CAD build for the part. Positions are in the model's coordinates, mm. A direction names the side the tool comes from. Coordinates: 2 decimals unless noted, no trailing zeros. Loops run counter-clockwise (first coordinate to the right, second up) from the corner with the lowest first, then second, coordinate; pieces in that order, holes last.
1) Saw through at B-B, the plane x = 113.5. Write the cut outline in (y, z), and give its area (3 significant figures).
2) Which spindle directions (+Z, -Z, +X, -X, +Y, -Y) get a long thin tool onto all of the face, cutting with end or side? Do faces 1 (the flat face through (109, 0, -8)), 2 (the flat face through (7, -5.634, -13)), 3 (the flat face through (184.81, 1.84, 1.58)). Say none if no direction does.
3) Saw through at A-A, the plane y = -3.5. Write the cut outline in (x, z), and give its area (3 significant figures).
4) Pin check, flat tips, straight feed: pin 1 Ø0.6 at (x, z) = (161.5, -15) entering from -Y; pin 2 Ø2 at (y, z) = (1, -14.5) entering from +X; pin 3 Ø3.5 at (x, z) = (64.5, -7.5) entering from +Y; pin 4 Ø5 at (x, y) = (129.5, 2.5) entering from +Z. Stop position of each tip, or through.
5) Saw through at C-C, the plane z = -6. Write the cut outline in (x, y).
6) Saw through at D-D, the plane x = 86.5. Write the cut outline in (y, z).
7) Two-plate mould, pull along X, no slides. Class faces 4 (the flat face through (203, -3, -16)), 5 (the flat face through (206, -1, -9)), 6 (the flat face through (15, -2, -10)): +X half, -X half, draft (parallel to the pull), parting line (faces both ways), or undercut.
8) Wall check: line 1 along X through (y, z) = (-1.5, -8.25); line 2 along Z through (x, y) = (152.5, 2.5); line 3 along Y through (x, z) = (93, -15). Give the ranges that are in metal, low to high.
```python
from build123d import *

# Parameters (mm, degrees)
EXTRUDE_PROFILE_DEPTH = 206
SKETCH6_W             = 185
SKETCH6_H             = 5.633658753
AIR_SPACE_DEPTH       = 45
SKETCH7_W             = 12
SKETCH7_H             = 3.530528437
TAB_CUTS_DEPTH        = 8.515248173
SKETCH8_W             = 15.5
SKETCH8_H             = 10
SKETCH8_W_2           = 6.5
CUT_EXTRUDE1_DEPTH    = 2


with BuildPart() as part:
    # Sketch1 → Extrude profile (new body)
    with BuildSketch(Plane(origin=(0, 0, 0), x_dir=(0, 0, -1), z_dir=(1, 0, 0))):
        Polygon((0, 1), (12, 1), (12, 4), (12, 5), (15, 5), (16, 4), (14, 4), (14, 2), (16, 2), (16, -5.633658753), (10.595371114, -5.633658753), (0, 0), (-3.531790371, 1.877886251), (-3.117271585, 2.657482703), align=None)
    extrude(amount=EXTRUDE_PROFILE_DEPTH)

    # Sketch6 → Air space (cut)
    with BuildSketch(Plane(origin=(0, 0, -16), x_dir=(-1, 0, 0), z_dir=(0, 0, -1))):
        with Locations((-107.5, -2.816829377)):
            Rectangle(SKETCH6_W, SKETCH6_H)
    extrude(amount=-AIR_SPACE_DEPTH, mode=Mode.SUBTRACT)

    # Sketch7 → Tab cuts (cut, through all)
    with BuildSketch(Plane(origin=(0, 0.779596452, -0.414518786), x_dir=(1, 0, 0), z_dir=(0, 0.882947593, -0.469471563))):
        with Locations((158.2, -2.234735781)):
            Rectangle(SKETCH7_W, SKETCH7_H)
        with Locations((88.1, -2.234735781)):
            Rectangle(SKETCH7_W, SKETCH7_H)
    extrude(amount=-TAB_CUTS_DEPTH, mode=Mode.SUBTRACT)

    # Sketch8 → Cut-Extrude1 (cut)
    with BuildSketch(Plane(origin=(0, 0, -16), x_dir=(-1, 0, 0), z_dir=(0, 0, -1))):
        with Locations((-198.25, 5)):
            Rectangle(SKETCH8_W, SKETCH8_H)
        with Locations((-70.55, 5)):
            Rectangle(SKETCH8_W_2, SKETCH8_H)
        with Locations((-79.45, 5)):
            Rectangle(SKETCH8_W_2, SKETCH8_H)
    extrude(amount=-CUT_EXTRUDE1_DEPTH, mode=Mode.SUBTRACT)


solid = part.part
```
Data:
1. outline: (0, -16) - (2, -16) - (2, -14) - (4, -14) - (4, -16) - (5, -15) - (5, -12) - (1, -12) - (1, 0) - (2.66, 3.12) - (1.88, 3.53) - (0, 0) - close
1. area: 30.8 mm2
2. face 1: +Z, -Z, -Y
2. face 2: +Z, -Z, +X, -X, -Y
2. face 3: +X, -X, +Y
3. outline: (0, -16) - (15, -16) - (15, -6.58) - (0, -6.58) - close; (200, -16) - (206, -16) - (206, -6.58) - (200, -6.58) - close
3. area: 198 mm2
4. pin 1: stops at y = 0
4. pin 2: stops at x = 206
4. pin 3: stops at y = 1
4. pin 4: stops at z = 3.53
5. outline: (0, -3.19) - (15, -3.19) - (15, 0) - (200, 0) - (200, -3.19) - (206, -3.19) - (206, 1) - (0, 1) - close
6. outline: (0, -16) - (2, -16) - (2, -14) - (4, -14) - (4, -16) - (5, -15) - (5, -12) - (1, -12) - (1, 0) - (0.22, 0.41) - (0, 0) - close
7. face 4: draft
7. face 5: +X half
7. face 6: undercut
8. line 1: x = 0 to 15, 200 to 206
8. line 2: z = -14 to -12
8. line 3: y = 0 to 2, 4 to 5
